Geometry: final body of the model. Coordinates: model frame, mm. Round coordinates to 2 decimals unless told otherwise and drop trailing zeros. Write each loop counter-clockwise with the first axis right and the second up, starting at its lowest first coordinate (ties: lowest second). Pieces come first, ordered by that corner, then holes. Notation, with made-up numbers: (35.5, 5.5) - (70.5, 5.5) arc R18 cw to (70.5, 38.5) - close; hole circle Ø6 at (-23.75, -3.5). An arc over 180 degrees is marked (long way). Write each question's results on one line, items separated by ' | '.
from build123d import *

# Parameters (mm, degrees)
SKETCH_1_R               = 11.1
EXTRUDE_1_DEPTH          = 72
SKETCH_2_W               = 62
SKETCH_2_H               = 70
SKETCH_2_H_2             = 67.94057246
CUT_EXTRUDE_1_DEPTH      = 70
EXTRUDE_2_DEPTH          = 62
EXTRUDE_3_DEPTH          = 62
CUT_EXTRUDE_3_DEPTH      = 130.811063026
CUT_EXTRUDE_3_DEPTH_BACK = 130.811063026
SKETCH_6_R               = 2.5
CUT_EXTRUDE_4_DEPTH      = 136.359998088
CUT_EXTRUDE_4_DEPTH_BACK = 136.359998088
SKETCH_7_W               = 62
SKETCH_7_H               = 120


with BuildPart() as part:
    # Sketch 1 → Extrude 1 (new body)
    with BuildSketch(Plane.XY):
        with BuildLine():
            Line((-15, 90), (-15, 0))
            ThreePointArc((-15, 0), (0, -15), (15, 0))
            Line((15, 0), (15, 90))
            ThreePointArc((15, 90), (0, 105), (-15, 90))
        make_face()
        Circle(SKETCH_1_R, mode=Mode.SUBTRACT)
        with Locations((0, 90)):
            Circle(SKETCH_1_R, mode=Mode.SUBTRACT)
    extrude(amount=EXTRUDE_1_DEPTH)

    # Sketch 2 → Cut-Extrude 1 (cut)
    with BuildSketch(Plane.ZY.offset(15)):
        with Locations((36, 80)):
            Rectangle(SKETCH_2_W, SKETCH_2_H)
        with Locations((36, 11.02971377)):
            Rectangle(SKETCH_2_W, SKETCH_2_H_2)
    extrude(amount=-CUT_EXTRUDE_1_DEPTH, mode=Mode.SUBTRACT)


with BuildPart() as cut_extrude_1_piece_1:
    # of the separate pieces the step leaves, piece 1, a body of its own (cut_extrude_1_pieces)
    add(part.part.solids().sort_by_distance((15, 0, 0))[0])



with BuildPart() as cut_extrude_1_piece_2:
    # of the separate pieces the step leaves, piece 2, a body of its own (cut_extrude_1_pieces)
    add(part.part.solids().sort_by_distance((15, 0, 67))[0])


with BuildPart() as cut_extrude_1_piece_1_1:
    add(cut_extrude_1_piece_1.part)

    add(cut_extrude_1_piece_2.part)  # Extrude 2 merges Cut-Extrude 1 piece 2
    # Sketch 4 → Extrude 2 (add)
    with BuildSketch(Plane(origin=(0, 0, 67), x_dir=(-1, 0, 0), z_dir=(0, 0, -1))):
        with BuildLine():
            Line((-4.490156776, 68.758657712), (15, 57.50601045))
            Line((15, 57.50601045), (36.319312502, 12.911360415))
            ThreePointArc((36.319312502, 12.911360415), (35.142094618, 9.577570071), (31.808304274, 10.754787955))
            Line((31.808304274, 10.754787955), (15, 45.913541163))
            Line((15, 45.913541163), (-9.509843224, 60.064305746))
            ThreePointArc((-9.509843224, 60.064305746), (-11.347175983, 66.921324953), (-4.490156776, 68.758657712))
        make_face()
    extrude(amount=EXTRUDE_2_DEPTH)

    # Sketch 5 → Extrude 3 (add)
    with BuildSketch(Plane(origin=(0, 0, 67), x_dir=(-1, 0, 0), z_dir=(0, 0, -1))):
        with BuildLine():
            Line((-30.017605928, 49.094069219), (-15, 60.919508718))
            Line((-15, 60.919508718), (12.5, 45.042376315))
            ThreePointArc((12.5, 45.042376315), (14.330127019, 38.212249296), (7.5, 36.382122277))
            Line((7.5, 36.382122277), (-15, 49.372503334))
            Line((-15, 49.372503334), (-27.615908762, 44.780688066))
            ThreePointArc((-27.615908762, 44.780688066), (-30.655195979, 45.913733224), (-30.017605928, 49.094069219))
        make_face()
    extrude(amount=EXTRUDE_3_DEPTH)

    # Sketch 6 → Cut-Extrude 3 (cut, two sides: drawn at the far end of the back side and taken through both)
    with BuildSketch(Plane(origin=(0, 0, 67), x_dir=(-1, 0, 0), z_dir=(0, 0, -1)).offset(-CUT_EXTRUDE_3_DEPTH_BACK)):
        with Locations(Location((-7, 64.411481729, 0), (0, 0, 90))):
            Circle(SKETCH_6_R)
        with Locations(Location((-11.650635095, 53.212249296, 0), (0, 0, 90))):
            Circle(SKETCH_6_R)
        with Locations(Location((10, 40.712249296, 0), (0, 0, 90))):
            Circle(SKETCH_6_R)
        with Locations(Location((10.320508076, 54.411481729, 0), (0, 0, 90))):
            Circle(SKETCH_6_R)
    extrude(amount=CUT_EXTRUDE_3_DEPTH + CUT_EXTRUDE_3_DEPTH_BACK, mode=Mode.SUBTRACT)

    # Sketch 7 → Cut-Extrude 4 (cut, two sides: drawn at the far end of the back side and taken through both)
    with BuildSketch(Plane.ZY.offset(15).offset(-CUT_EXTRUDE_4_DEPTH_BACK)):
        with Locations((36, 45)):
            Rectangle(SKETCH_7_W, SKETCH_7_H)
    extrude(amount=CUT_EXTRUDE_4_DEPTH + CUT_EXTRUDE_4_DEPTH_BACK, mode=Mode.SUBTRACT)


with BuildPart() as cut_extrude_4_piece_1:
    # of the separate pieces the step leaves, piece 1, a body of its own (cut_extrude_4_pieces)
    add(cut_extrude_1_piece_1_1.part.solids().sort_by_distance((-15, 90, 5))[0])


with BuildPart() as cut_extrude_4_piece_2:
    # of the separate pieces the step leaves, piece 2, a body of its own (cut_extrude_4_pieces)
    add(cut_extrude_1_piece_1_1.part.solids().sort_by_distance((15, 0, 67))[0])


solid = cut_extrude_4_piece_2.part
Q1. Mould query, pull axis Y, two halves, no side actions, for faces 1 (the cylindrical face through (0, 105, 69)), 2 (the flat face through (-15, 46, 69)), 3 (the cylindrical face through (5.97, 9.36, 69.46)). Classes: pulls with the +Y half, pulls with the -Y half, needs draft (parallel to the pull), parting line crosses it, or undercut.
Answer block:
face 1: pulls with the +Y half | face 2: needs draft | face 3: undercut
Q2. Pin query (flat end, axial travel): pin 1 (4.5 mm diameter, centred on x = -10.32, y = 54.41, fed in from -Z); pin 2 (1 mm diameter, centred on x = 10.5, z = 68.5, fed in from +Y); pin 3 (6 mm diameter, centred on x = -10, y = 40.71, fed in from +Z); pin 4 (1 mm diameter, centred on y = 92.5, z = 70, fed in from +X). Return the tip coordinate at first contact, or that it passes through.
Answer block:
pin 1: through | pin 2: y = 101.18 | pin 3: z = 72 | pin 4: x = 14.87
Q3. Section query D-D, the plane z = 70.4. Return loops of the section in (x, y), plus the area to 3 significant figures.
Answer block:
outline: (-15, 0) arc R15 ccw to (15, 0) - (15, 90) arc R15 ccw to (-15, 90) - close; hole circle Ø5 at (-10.32, 54.41); hole circle Ø5 at (-10, 40.71); hole circle Ø22.2 at (0, 0); hole circle Ø22.2 at (0, 90); hole circle Ø5 at (7, 64.41); hole circle Ø5 at (11.65, 53.21) | area: 2,550 mm2
Q4. Ray query, line 1 along Y through (x, z) = (-2, 67.3); line 2 along Y through (x, z) = (-4, 67.5); line 3 along X through (y, z) = (0, 70.1). Return the intervals inside material, ascending.
Answer block:
line 1: -14.87 to -10.92, 10.92 to 79.08, 100.92 to 104.87 | line 2: -14.46 to -10.35, 10.35 to 79.65, 100.35 to 104.46 | line 3: -15 to -11.1, 11.1 to 15
Q5. Section query A-A, the plane y = 6.5. Return loops of the section in (x, z).
Answer block:
outline: (-15, 67) - (-9, 67) - (-9, 72) - (-15, 72) - close; (9, 67) - (15, 67) - (15, 72) - (9, 72) - close
Q6. Section query C-C, the plane x = -2. Return loops of the section in (y, z).
Answer block:
outline: (-14.87, 67) - (-10.92, 67) - (-10.92, 72) - (-14.87, 72) - close; (10.92, 67) - (79.08, 67) - (79.08, 72) - (10.92, 72) - close; (100.92, 67) - (104.87, 67) - (104.87, 72) - (100.92, 72) - close
Q7. Section query B-B, the plane x = 7. Return loops of the section in (y, z).
Answer block:
outline: (-13.27, 67) - (-8.61, 67) - (-8.61, 72) - (-13.27, 72) - close; (8.61, 67) - (61.91, 67) - (61.91, 72) - (8.61, 72) - close; (66.91, 67) - (81.39, 67) - (81.39, 72) - (66.91, 72) - close; (98.61, 67) - (103.27, 67) - (103.27, 72) - (98.61, 72) - close
